Geometry: see drawing. Coordinates: mm, zero at the bounding-box minimum. A direction names the side the tool comes from. Round coordinates to 2 decimals unless told otherwise and drop trailing zeros. Loops run counter-clockwise (first coordinate to the right, second up) from the corner with the lowest first, then second, coordinate; pieces in that order, holes last.
(1) Cut plane D-D, the plane x = 2.75. Output: boundary loops of the cut face in (y, z), and give its area (3 significant figures).
(2) Line query: line 1 (X direction, y = 4, z = 8); line 2 (Z direction, x = 19.25, y = 8.25); line 3 (Y direction, x = 18.5, z = 12.75). Output: solid intervals per line, ascending.
(3) Cut plane A-A, the plane y = 8. Output: boundary loops of the cut face in (x, z), and give its area (4 significant figures).
(4) Cut plane C-C, the plane x = 19. Output: boundary loops of the cut face in (y, z), and give its area (3 significant figures).
(5) Access query for the marked faces 1 and 2. Directions: +Z, -Z, +X, -X, +Y, -Y. A direction counts if a zero-diameter tool reaches every point of the face in a straight line with its end or side. Return the directions, or none.
(6) First-contact query: pin 1 Ø8 at (x, z) = (13.5, 10) entering from -Y; pin 2 Ø5 at (x, y) = (5, 5.5) entering from -Z; pin 3 Ø6 at (x, z) = (14.5, 2.5) entering from -Y; pin 4 Ø4 at (x, z) = (7, 5.5) entering from +Y. Flat tips, straight axial feed; report the tip coordinate or a pass-through.
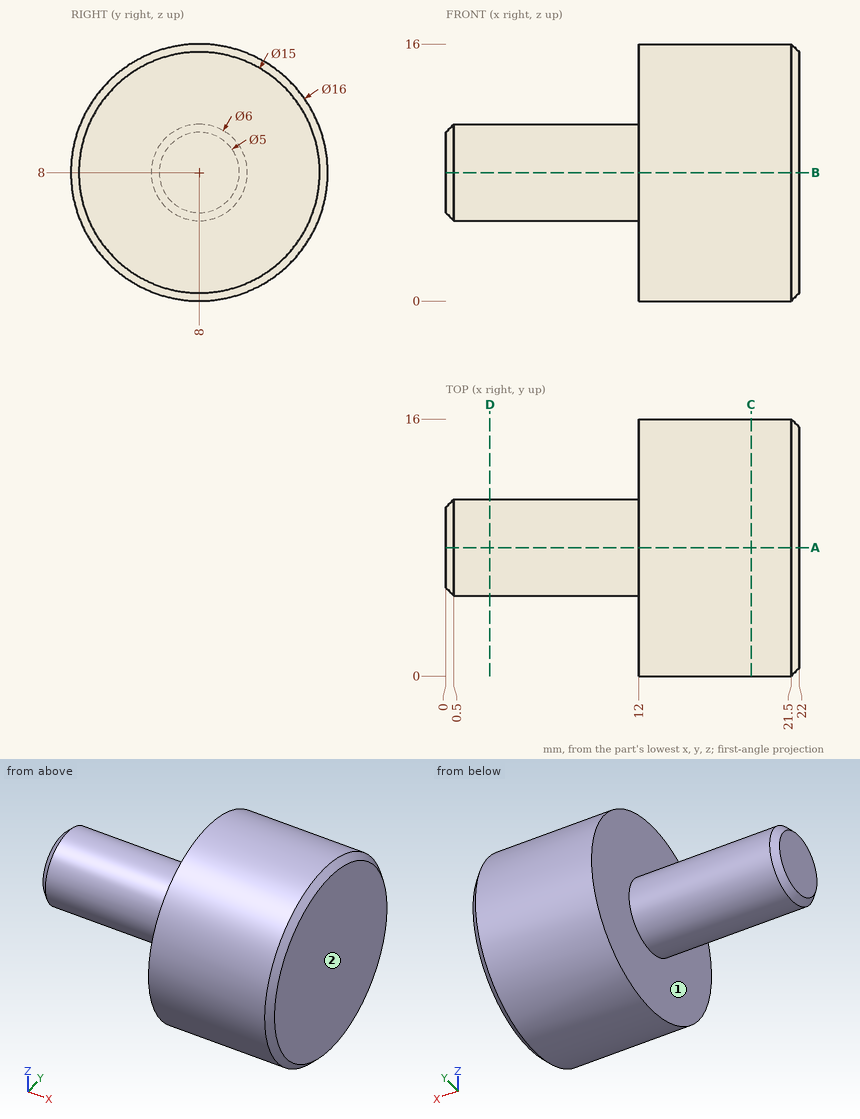
Reported:
1. outline: circle Ø6 at (8, 8)
1. area: 28.3 mm2
2. line 1: x = 12 to 22
2. line 2: z = 0 to 16
2. line 3: y = 1.56 to 14.44
3. outline: (0, 5.5) - (0.5, 5) - (12, 5) - (12, 0) - (21.5, 0) - (22, 0.5) - (22, 15.5) - (21.5, 16) - (12, 16) - (12, 11) - (0.5, 11) - (0, 10.5) - close
3. area: 231.5 mm2
4. outline: circle Ø16 at (8, 8)
4. area: 201 mm2
5. face 1: -X
5. face 2: +Z, -Z, +X, +Y, -Y
6. pin 1: stops at y = 0
6. pin 2: stops at z = 5
6. pin 3: stops at y = 0.4
6. pin 4: stops at y = 10.96
